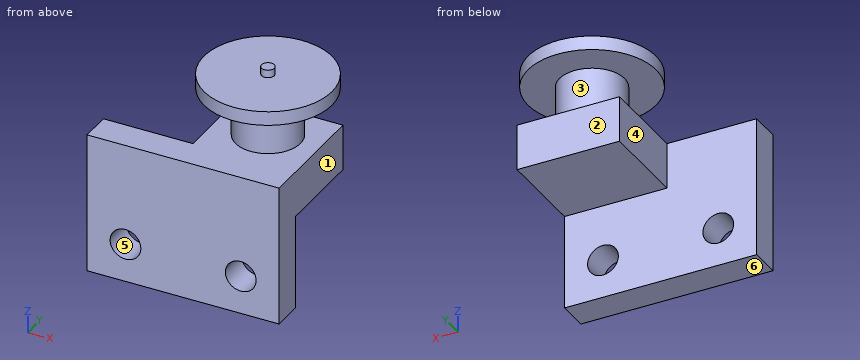
```python
from build123d import *

# Parameters (mm, degrees)
F0_W      = 100
F0_H      = 35
F1_DEPTH  = 18
F3_D      = 12
F4_R      = 12.7
F5_DEPTH  = 19
F6_R      = 25
F6_R_2    = 12.7
F7_DEPTH  = 5.5
F8_R      = 2.5
F9_DEPTH  = 3
F10_W     = 100
F10_H     = 57
F10_H_2   = 18
F11_DEPTH = 12
F12_W     = 30
F12_H     = 35
F13_DEPTH = 25
F14_W     = 30
F14_H     = 75
F15_DEPTH = 25
F16_W     = 75
F16_H     = 55
F17_DEPTH = 12
F18_W     = 40
F18_H     = 20
F19_DEPTH = 25
F21_D     = 12


with BuildPart() as f1:
    # F0 (on Top) → F1 (new body)
    with BuildSketch(Plane.XY):
        Rectangle(F0_W, F0_H)
    extrude(amount=-F1_DEPTH)

    # F3 (through all)
    with Locations(Plane.XY):
        with Locations((-38, 0), (38, 0)):
            Hole(F3_D / 2)

    # F4 (on face) → F5 (join)
    with BuildSketch(Plane.XY):
        Circle(F4_R)
    extrude(amount=F5_DEPTH)

    # F6 (on face) → F7 (join)
    with BuildSketch(Plane.XY.offset(19)):
        Circle(F6_R)
        Circle(F6_R_2, mode=Mode.SUBTRACT)
        Circle(F6_R_2)
    extrude(amount=F7_DEPTH)

    # F8 (on face) → F9 (join)
    with BuildSketch(Plane.XY.offset(24.5)):
        Circle(F8_R)
    extrude(amount=F9_DEPTH)

    # F10 (on face) → F11 (join)
    with BuildSketch(Plane.XZ.offset(17.5)):
        with Locations((0, -46.5)):
            Rectangle(F10_W, F10_H)
        with Locations((0, -9)):
            Rectangle(F10_W, F10_H_2)
    extrude(amount=F11_DEPTH)

    # F12 (on face) → F13 (cut)
    with BuildSketch(Plane(origin=(0, 0, -18), x_dir=(1, 0, 0), z_dir=(0, 0, -1))):
        with Locations((35, 0)):
            Rectangle(F12_W, F12_H)
        with Locations((-35, 0)):
            Rectangle(F12_W, F12_H)
    extrude(amount=-F13_DEPTH, mode=Mode.SUBTRACT)

    # F14 (on face) → F15 (cut)
    with BuildSketch(Plane(origin=(0, -17.5, 0), x_dir=(-1, 0, 0), z_dir=(0, 1, 0))):
        with Locations((-35, -37.5)):
            Rectangle(F14_W, F14_H)
        with Locations((35, -37.5)):
            Rectangle(F14_W, F14_H)
    extrude(amount=-F15_DEPTH, mode=Mode.SUBTRACT)

    # F16 (on face) → F17 (join)
    with BuildSketch(Plane.XZ.offset(29.5)):
        with Locations((-17.5, -27.5)):
            Rectangle(F16_W, F16_H)
    extrude(amount=-F17_DEPTH)

    # F18 (on face) → F19 (cut)
    with BuildSketch(Plane.XZ.offset(29.5)):
        with Locations((0, -65)):
            Rectangle(F18_W, F18_H)
    extrude(amount=-F19_DEPTH, mode=Mode.SUBTRACT)

    # F21 (through all)
    with Locations(Plane(origin=(0, -17.5, 0), x_dir=(-1, 0, 0), z_dir=(0, 1, 0))):
        with Locations((-5, -40), (40, -40)):
            Hole(F21_D / 2)


solid = f1.part
```
Verification items for the finished model (mm, model axes). Face numbers are marked on the shaded views. A direction names the side the tool comes from. Coordinates: 2 decimals unless noted, no trailing zeros. Order: outer loops, then holes, each group sorted by start corner. A loop starts at its lowest first (then second) coordinate and runs counter-clockwise, first axis right, second up. Notation, with made-up numbers: (38.5, 13.25) -> (75.5, 13.25) arc R22 cw to (75.5, 20.25) -> close; hole circle Ø9 at (-24, -34.5). An arc over 180 degrees is marked (long way). Put each result on its own line as item: value. Start each with the question number.
1) Cross-section at B-B (z = -40). Enter the section's corners in (x, y), plus the area to 3 significant figures.
2) Cross-section at C-C (y = 0). Enter the section's corners in (x, z).
3) Cross-section at D-D (z = -2). Enter the section's corners in (x, y).
4) Go/stop test with flat-tipped pins: pin 1 (8 mm diameter, centred on y = 19, z = -20.5, fed in from +X); pin 2 (1.5 mm diameter, centred on x = -22, y = 7.5, fed in from -Z); pin 3 (14 mm diameter, centred on x = -40, z = -40, fed in from +Y). Record where each tip stops, or that it passes through.
5) Release check for a two-part mould opening along Z. For the marked faces 4, 5 and 6 record: pulls with the +Z half, pulls with the -Z half, needs draft (parallel to the pull), parting line crosses it, or undercut.
6) Cross-section at A-A (x = -40). Enter the section's corners in (y, z).
7) Tool access check on the marked faces 1, 2 and 3. Record the directions out of +Z, -Z, +X, -X, +Y, -Y that give a thin tool (end or side, any length) a straight path to the whole face; none if there is none.
8) Material ranges on L1, parallel to Z at x = -40, y = -20; L2, parallel to Z at x = -19, y = -11; L3, parallel to X at y = -14, z = -16.5, recorded low to high.
Geometry check:
1. outline: (-55, -29.5) -> (-46, -29.5) -> (-46, -17.5) -> (-55, -17.5) -> close; (-34, -29.5) -> (-1, -29.5) -> (-1, -17.5) -> (-34, -17.5) -> close; (11, -29.5) -> (20, -29.5) -> (20, -17.5) -> (11, -17.5) -> close
1. area: 612 mm^2
2. outline: (-25, 19) -> (-12.7, 19) -> (-12.7, 0) -> (-20, 0) -> (-20, -18) -> (20, -18) -> (20, 0) -> (12.7, 0) -> (12.7, 19) -> (25, 19) -> (25, 24.5) -> (2.5, 24.5) -> (2.5, 27.5) -> (-2.5, 27.5) -> (-2.5, 24.5) -> (-25, 24.5) -> close
3. outline: (-55, -29.5) -> (20, -29.5) -> (20, 17.5) -> (-20, 17.5) -> (-20, -17.5) -> (-55, -17.5) -> close
4. pin 1: stops at x = 20
4. pin 2: stops at z = 19
4. pin 3: stops at y = -17.5
5. face 4: needs draft
5. face 5: undercut
5. face 6: pulls with the -Z half
6. outline: (-29.5, -55) -> (-17.5, -55) -> (-17.5, -46) -> (-29.5, -46) -> close; (-29.5, -34) -> (-17.5, -34) -> (-17.5, 0) -> (-29.5, 0) -> close
7. face 1: -Z, +X, +Y, -Y
7. face 2: -Z, +X, -X, +Y
7. face 3: none
8. L1: z = -55 to -46, -34 to 0
8. L2: z = -18 to 0, 19 to 24.5
8. L3: x = -20 to 20
